```python
from build123d import *

# Parameters (mm, degrees)
F0_W     = 77.8612360591
F0_H     = 53.5927973688
F1_DEPTH = 31.75
F2_T     = -2.54
F3_R     = 5.08


with BuildPart() as f1:
    # F0 (on Top) → F1 (new body)
    with BuildSketch(Plane.XY):
        with Locations((40.8265881124, -26.7963986844)):
            Rectangle(F0_W, F0_H)
    extrude(amount=F1_DEPTH)

    # F2
    f2_openings = [f1.faces().sort_by_distance(p)[0] for p in [
        (40.826588, -26.796399, 31.75),
    ]]
    offset(amount=F2_T, openings=f2_openings)

    # F3
    f3_edges = [f1.edges().sort_by_distance(p)[0] for p in [
        (1.89597, 0, 15.875),
        (79.757206, 0, 15.875),
        (79.757206, -53.592797, 15.875),
        (1.89597, -53.592797, 15.875),
        (4.43597, -51.052797, 17.145),
        (4.43597, -2.54, 17.145),
        (77.217206, -2.54, 17.145),
        (77.217206, -51.052797, 17.145),
    ]]
    fillet(f3_edges, radius=F3_R)


solid = f1.part
```
Input: part model. Units: mm. Frame: model coordinates. A direction names the side the tool comes from. Coordinates: 2 decimals unless noted, no trailing zeros. Write each loop counter-clockwise with the first axis right and the second up, starting at its lowest first coordinate (ties: lowest second). Pieces come first, ordered by that corner, then holes.
1) Section A-A on y = -15.5. Output: boundary loops of the cut face in (x, z), and give its area (3 significant figures).
2) Material intervals for line 1 along X through (y, z) = (-31.5, 24.5); line 2 along Y through (x, z) = (55.5, 15.5); line 3 along Z through (x, y) = (25.5, -15.5), sorted ascending.
3) Mould query, pull axis Y, two halves, no side actions, for faces 3 (the cylindrical face through (3.345, -52.065, 16.097)), 4 (the cylindrical face through (78.31, -1.53, 16.1)), 5 (the flat face through (1.896, -27, 16)), 6 (the cylindrical face through (5.885, -49.525, 16.941)). Classes: pulls with the +Y half, pulls with the -Y half, needs draft (parallel to the pull), parting line crosses it, or undercut.
4) Set-up query: faces 1 (the flat face through (40, 0, 16)), 2 (the cylindrical face through (5.88, -4.07, 16.94)). Return all of +Z, -Z, +X, -X, +Y, -Y with unobstructed straight access to the full face (end or side cutting, diameter ignored); none if empty.
5) Section B-B on x = 68.5. Output: boundary loops of the cut face in (y, z).
6) Section C-C on z = 24. Output: boundary loops of the cut face in (x, y).
Check result:
1. outline: (1.9, 0) - (79.76, 0) - (79.76, 31.75) - (77.22, 31.75) - (77.22, 2.54) - (4.44, 2.54) - (4.44, 31.75) - (1.9, 31.75) - close
1. area: 346 mm2
2. line 1: x = 1.9 to 4.44, 77.22 to 79.76
2. line 2: y = -53.59 to -51.05, -2.54 to 0
2. line 3: z = 0 to 2.54
3. face 3: pulls with the -Y half
3. face 4: pulls with the +Y half
3. face 5: needs draft
3. face 6: undercut
4. face 1: +Z, -Z, +X, -X, +Y
4. face 2: +Z
5. outline: (-53.59, 0) - (0, 0) - (0, 31.75) - (-2.54, 31.75) - (-2.54, 2.54) - (-51.05, 2.54) - (-51.05, 31.75) - (-53.59, 31.75) - close
6. outline: (1.9, -48.51) arc R5.08 ccw to (6.98, -53.59) - (74.68, -53.59) arc R5.08 ccw to (79.76, -48.51) - (79.76, -5.08) arc R5.08 ccw to (74.68, 0) - (6.98, 0) arc R5.08 ccw to (1.9, -5.08) - close; hole (4.44, -45.97) arc R5.08 ccw to (9.52, -51.05) - (72.14, -51.05) arc R5.08 ccw to (77.22, -45.97) - (77.22, -7.62) arc R5.08 ccw to (72.14, -2.54) - (9.52, -2.54) arc R5.08 ccw to (4.44, -7.62) - close
